The listing builds one solid part. Answer for the finished solid, in the listing's coordinates (mm). A direction names the side the tool comes from. Round coordinates to 2 decimals unless told otherwise and drop trailing zeros. Write each loop counter-clockwise with the first axis right and the second up, starting at its lowest first coordinate (ties: lowest second). Pieces come first, ordered by that corner, then holes. Notation, with made-up numbers: (86.25, -16) - (93.25, -16) arc R21 cw to (93.25, -2) - close; hole circle Ø5 at (-6, 43.25). An arc over 180 degrees is marked (long way). Return JSON: item names as keys, results as strings. Group by question number.
(1) Determine the mould class of faces 1 (the flat face through (0.521, 3.719, 3.976)), 2 (the flat face through (1.612, -3.316, -1.016)), 3 (the flat face through (2.726, 0.322, -3.286)) for opening direction Z: +Z half, -Z half, draft (parallel to the pull), parting line (faces both ways), or undercut.
(2) Find the intervals of material crossed by line 1 along Y through (x, z) = (11.5, 0.5); line 2 along Y through (x, z) = (2, 3.5), in increasing order. Write a range as [from, to].
(3) Section A-A, the plane x = 4.5 is taken. Write down the section's boundary in (y, z), then the cut area to 3 significant figures.
(4) Which of the six approach directions +Z, -Z, +X, -X, +Y, -Y give full straight-line access (tool end or side, diameter ignored) to faces 4 (the flat face through (2.72, 1.75, 2.8)), 5 (the flat face through (1.61, -0.78, -3.38)), 6 (the flat face through (0.52, 1.58, -5.21))?
(5) Each of these flat-tipped pins is pushed along its axis until it touches: pin 1 (1.4 mm diameter, centred on x = 7, y = 0, fed in from -Z); pin 2 (6 mm diameter, centred on x = 6, y = -2, fed in from -Z); pin 3 (0.9 mm diameter, centred on x = 6, z = 0.5, fed in from +Y). Where does it stop, or does it pass through?
Autodesk Inventor part; units mm, degrees
ref_plane "YZ Plane" through (0, 0, 0) normal (1, 0, 0) x (0, 1, 0)
ref_plane "XZ Plane" through (0, 0, 0) normal (0, 1, 0) x (-1, 0, 0)
ref_plane "XY Plane" through (0, 0, 0) normal (0, 0, 1) x (1, 0, 0)
sketch "Sketch6" plane through (0, 0, 0) normal (1, 0, 0) x (0, 1, 0)
  line L0 (5.2569, 0.1572) -> (4.6312, -2.4922)
  line L1 (4.6312, -2.4922) -> (2.7646, -4.4739)
  line L2 (2.7646, -4.4739) -> (0.1572, -5.2569)
  line L3 (0.1572, -5.2569) -> (-2.4922, -4.6312)
  line L4 (-2.4922, -4.6312) -> (-4.4739, -2.7646)
  line L5 (-4.4739, -2.7646) -> (-5.2569, -0.1572)
  line L6 (-5.2569, -0.1572) -> (-4.6312, 2.4922)
  line L7 (-4.6312, 2.4922) -> (-2.7646, 4.4739)
  line L8 (-2.7646, 4.4739) -> (-0.1572, 5.2569)
  line L9 (-0.1572, 5.2569) -> (2.4922, 4.6312)
  line L10 (2.4922, 4.6312) -> (4.4739, 2.7646)
  line L11 (4.4739, 2.7646) -> (5.2569, 0.1572)
  point P0 (0, 0)
  point P1 (0, 0)
  dimension "d27" = 5.08
extrude "Extrusion2" add sketch "Sketch6" along normal blind 6.096 draft -45
sketch "Sketch7" plane through (0, 2.4922, 4.6312) normal (0.7071068, 0.484827, 0.5147259) x (0, 0.7279324, -0.6856489)
  line L0 (0, 0) -> (2.7224, 0)
  line L1 (0, 0) -> (2.7224, 0)
  line L2 (2.7224, 0) -> (1.3511, -7.2372)
  line L3 (2.7224, 0) -> (1.3612, -7.1842)
  line L4 (1.3511, -7.2372) -> (0, 0)
  point P0 (1.3612, -3.5921)
  dimension "d38" = 0
  dimension "d30" = 7.366
extrude "Extrusion3" add sketch "Sketch7" along normal blind 1.27 draft -10
sketch "Sketch8" plane through (0, 0, 0) normal (-1, 0, 0) x (0, 0, 1)
  line L0 (-0.889, -0.889) -> (0.889, -0.889)
  line L1 (0.889, -0.889) -> (0.889, 0.889)
  line L2 (0.889, 0.889) -> (-0.889, 0.889)
  line L3 (-0.889, 0.889) -> (-0.889, -0.889)
  line L4 (-0.889, -0.889) -> (0.889, 0.889) construction
  line L5 (0.889, -0.889) -> (-0.889, 0.889) construction
  point P0 (0, 0)
  dimension "d33" = 1.778
  dimension "d34" = 1.778
extrude "Extrusion4" add sketch "Sketch8" against normal blind 12.7
sketch "Sketch9" plane through (12.7, 0, 0) normal (1, 0, 0) x (0, 0, 1)
  circle A0 centre (0, 0) radius 0.0758
  point P0 (0, 0)
extrude "Extrusion5" add sketch "Sketch9" along normal blind 0.0254
pattern_circular "Circular Pattern1" count 6 over 360 about axis through (12.7, 0, 0) along (1, 0, 0) of "Extrusion3"
properties part number "RotateGear"
Working result:
{
 "1": {"face 1": "+Z half", "face 2": "undercut", "face 3": "-Z half"},
 "2": {"line 1": "y = [-0.89, 0.89]", "line 2": "y = [-1.93, -0.19], [2.15, 3.4]"},
 "3": {"outline": "(-2.35, 0.37) - (-0.89, 0.03) - (-0.89, -0.71) - (-1.75, -1.61) - (-1.5, -1.85) - (-0.6, -0.89) - (0.1, -0.89) - (0.52, -2.32) - (0.86, -2.22) - (0.45, -0.89) - (0.89, -0.89) - (0.89, -0.37) - (2.27, -0.71) - (2.35, -0.37) - (0.89, -0.03) - (0.89, 0.71) - (1.75, 1.61) - (1.5, 1.85) - (0.6, 0.89) - (-0.1, 0.89) - (-0.52, 2.32) - (-0.86, 2.22) - (-0.45, 0.89) - (-0.89, 0.89) - (-0.89, 0.37) - (-2.27, 0.71) - close", "area": "5.98 mm^2"},
 "4": {"face 4": "+Z, +X", "face 5": "-Z, +X", "face 6": "-Z, -X, +Y"},
 "5": {"pin 1": "stops at z = -0.89", "pin 2": "stops at z = -3.21", "pin 3": "stops at y = 0.89"}
}
